```python
from build123d import *

# Parameters (mm, degrees)
SKETCH1_W          = 73
SKETCH1_H          = 60
PLATE_DEPTH        = 14
SKETCH2_R          = 2.5
CUT_EXTRUDE4_DEPTH = 16
FILLET1_R          = 10
FILLET2_R          = 10
FILLET3_R          = 10
FILLET4_R          = 10


with BuildPart() as part:
    # Sketch1 → Plate (new body)
    with BuildSketch(Plane.XY):
        Rectangle(SKETCH1_W, SKETCH1_H)
    extrude(amount=PLATE_DEPTH)

    # Sketch2 → Cut-Extrude4 (cut)
    with BuildSketch(Plane.XY.offset(14)):
        with Locations((-30.310889135, 17)):
            Circle(SKETCH2_R)
        with Locations((30.310889135, 17)):
            Circle(SKETCH2_R)
        with Locations((30.310889135, -18)):
            Circle(SKETCH2_R)
        with Locations((-30.310889135, -18)):
            Circle(SKETCH2_R)
    extrude(amount=-CUT_EXTRUDE4_DEPTH, mode=Mode.SUBTRACT)

    # Fillet1
    fillet1_edges = [part.edges().sort_by_distance(p)[0] for p in [
        (36.5, -30, 7),
    ]]
    fillet(fillet1_edges, radius=FILLET1_R)

    # Fillet2
    fillet2_edges = [part.edges().sort_by_distance(p)[0] for p in [
        (36.5, 30, 7),
    ]]
    fillet(fillet2_edges, radius=FILLET2_R)

    # Fillet3
    fillet3_edges = [part.edges().sort_by_distance(p)[0] for p in [
        (-36.5, 30, 7),
    ]]
    fillet(fillet3_edges, radius=FILLET3_R)

    # Fillet4
    fillet4_edges = [part.edges().sort_by_distance(p)[0] for p in [
        (-36.5, -30, 7),
    ]]
    fillet(fillet4_edges, radius=FILLET4_R)


solid = part.part
```
Check sheet for the modelled part. Datum: model origin and axes. Units: mm. Give positions to 0.01 mm unless a question says otherwise; leave off trailing zeros. Write each loop counter-clockwise with the first axis right and the second up, starting at its lowest first coordinate (ties: lowest second). Pieces come first, ordered by that corner, then holes. Notation, with made-up numbers: (88, 66) - (143, 66) arc R37 ccw to (143, 105) - close; hole circle Ø4 at (84, 12.5). An arc over 180 degrees is marked (long way). Answer as a JSON object with one key per item and string values. Group by question number.
1) Sectioned sample at D-D (y = 24.5). Record the cut outline in (x, z), then the cut area to 3 significant figures.
2) Thickness scan on probe 1 along Y at (x, z) = (29, 8); probe 2 along X at (y, z) = (15, 10); probe 3 along X at (y, z) = (24.5, 12). Record the ranges inside material, lowest first. Write a range as from..to.
3) Sectioned sample at B-B (y = 17). Record the cut outline in (x, z).
4) Sectioned sample at C-C (y = -16.5). Record the cut outline in (x, z), then the cut area to 3 significant figures.
5) Release check for a two-part mould opening along Y. For faces 1 (the face through (-36.5, 0, 7)), 2 (the face through (-27.926, 17.751, 7.098)), 3 (the face through (27.813, -17.89, 7.098)), 4 (the face through (33.49, -27.15, 7.1)) record: pulls with the +Y half, pulls with the -Y half, needs draft (parallel to the pull), parting line crosses it, or undercut.
6) Sectioned sample at A-A (z = 3.5). Record the cut outline in (x, y), then the cut area to 3 significant figures.
Geometry results:
{
 "1": {"outline": "(-35.43, 0) - (35.43, 0) - (35.43, 14) - (-35.43, 14) - close", "area": "992 mm^2"},
 "2": {"probe 1": "y = -29.68..-20.13, -15.87..14.87, 19.13..29.68", "probe 2": "x = -36.5..-31.81, -28.81..28.81, 31.81..36.5", "probe 3": "x = -35.43..35.43"},
 "3": {"outline": "(-36.5, 0) - (-32.81, 0) - (-32.81, 14) - (-36.5, 14) - close; (-27.81, 0) - (27.81, 0) - (27.81, 14) - (-27.81, 14) - close; (32.81, 0) - (36.5, 0) - (36.5, 14) - (32.81, 14) - close"},
 "4": {"outline": "(-36.5, 0) - (-32.31, 0) - (-32.31, 14) - (-36.5, 14) - close; (-28.31, 0) - (28.31, 0) - (28.31, 14) - (-28.31, 14) - close; (32.31, 0) - (36.5, 0) - (36.5, 14) - (32.31, 14) - close", "area": "910 mm^2"},
 "5": {"face 1": "needs draft", "face 2": "undercut", "face 3": "undercut", "face 4": "pulls with the -Y half"},
 "6": {"outline": "(-36.5, -20) arc R10 ccw to (-26.5, -30) - (26.5, -30) arc R10 ccw to (36.5, -20) - (36.5, 20) arc R10 ccw to (26.5, 30) - (-26.5, 30) arc R10 ccw to (-36.5, 20) - close; hole circle Ø5 at (-30.31, -18); hole circle Ø5 at (-30.31, 17); hole circle Ø5 at (30.31, -18); hole circle Ø5 at (30.31, 17)", "area": "4,220 mm^2"}
}
